from build123d import *

# Parameters (mm, degrees)
F0_R     = 25
F1_DEPTH = 3


with BuildPart() as f1:
    # F0 (on Top) → F1 (new body)
    with BuildSketch(Plane.XY):
        with BuildLine():
            ThreePointArc((125, 100), (117.67767, 117.67767), (100, 125))
            Line((100, 125), (-100, 125))
            ThreePointArc((-100, 125), (-117.67767, 117.67767), (-125, 100))
            Line((-125, 100), (-125, -100))
            ThreePointArc((-125, -100), (-117.67767, -117.67767), (-100, -125))
            Line((-100, -125), (100, -125))
            ThreePointArc((100, -125), (117.67767, -117.67767), (125, -100))
            Line((125, -100), (125, 100))
        make_face()
        with Locations((-56.568542, -56.568542)):
            Circle(F0_R, mode=Mode.SUBTRACT)
        with Locations((0, -80)):
            Circle(F0_R, mode=Mode.SUBTRACT)
        with Locations((56.568542, -56.568542)):
            Circle(F0_R, mode=Mode.SUBTRACT)
        with Locations((-80, 0)):
            Circle(F0_R, mode=Mode.SUBTRACT)
        with Locations((-56.568542, 56.568542)):
            Circle(F0_R, mode=Mode.SUBTRACT)
        Circle(F0_R, mode=Mode.SUBTRACT)
        with Locations((56.568542, 56.568542)):
            Circle(F0_R, mode=Mode.SUBTRACT)
        with Locations((80, 0)):
            Circle(F0_R, mode=Mode.SUBTRACT)
        with Locations((0, 80)):
            Circle(F0_R, mode=Mode.SUBTRACT)
    extrude(amount=F1_DEPTH)


solid = f1.part
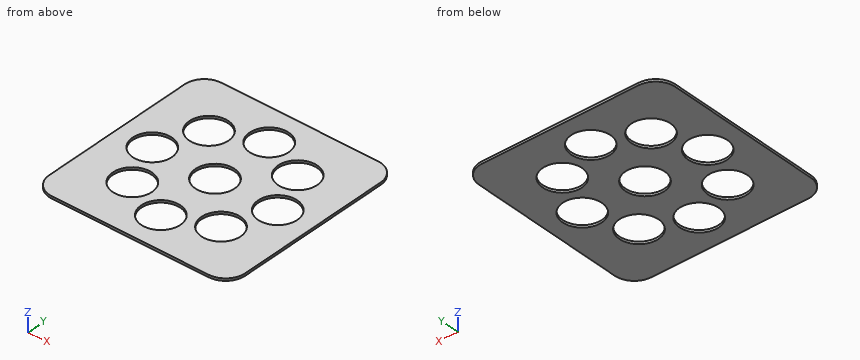
Design review of the part built by this model. Coordinates are the model's own, in mm. Give positions to 0.01 mm unless a question says otherwise; leave off trailing zeros. Order: outer loops, then holes, each group sorted by start corner. A loop starts at its lowest first (then second) coordinate and runs counter-clockwise, first axis right, second up.
1. Add section C-C, the plane z = 0.5. State how many separate pieces and enclosed holes the cut face has, then the cut area to 3 significant figures.
Solution:
separate pieces: 1
enclosed holes: 9
area: 44,300 mm2
2. Add section A-A, the plane x = 0. State the section outline as (y, z) points, then the cut area to 3 significant figures.
Solution:
outline: (-125, 0) - (-105, 0) - (-105, 3) - (-125, 3) - close; (-55, 0) - (-25, 0) - (-25, 3) - (-55, 3) - close; (25, 0) - (55, 0) - (55, 3) - (25, 3) - close; (105, 0) - (125, 0) - (125, 3) - (105, 3) - close
area: 300 mm2
3. For pin 1 Ø6 at (x, y) = (-14.5, -39) entering from -Z, flat-tipped, find the tip position at first contact; note if it passes through.
Solution:
pin 1: stops at z = 0
4. Add section D-D, the plane y = 86.5. State the section outline as (x, z) points, then the cut area to 3 significant figures.
Solution:
outline: (-125, 0) - (-24.14, 0) - (-24.14, 3) - (-125, 3) - close; (24.14, 0) - (125, 0) - (125, 3) - (24.14, 3) - close
area: 605 mm2
5. To check wall thickness, follow L1, parallel to Y at x = 0, z = 2.4; L2, parallel to X at y = -0.5, z = 0.4 (3 decimals); L3, parallel to X at y = 14, z = 0.5. State the ranges of each line that lie inside material, in increasing order.
Solution:
L1: y = -125 to -105, -55 to -25, 25 to 55, 105 to 125
L2: x = -125 to -104.995, -55.005 to -24.995, 24.995 to 55.005, 104.995 to 125
L3: x = -125 to -100.71, -59.29 to -20.71, 20.71 to 59.29, 100.71 to 125
